Part model, mm, in its own coordinate system. A direction names the side the tool comes from. Give positions to 0.01 mm unless a question says otherwise; leave off trailing zeros. Order: outer loops, then holes, each group sorted by start corner. A loop starts at its lowest first (then second) coordinate and runs counter-clockwise, first axis right, second up. Notation, with made-up numbers: (87, -39.5) -> (125, -39.5) arc R19 cw to (125, -3.5) -> close; hole circle Ø1 at (-19.5, 22). An arc over 180 degrees is marked (long way). Write item = value, one per line. Start each with the question number.
Item 1: Band-saw the part on A-A on y = 37.5. Write the cut outline in (x, z), plus the area to 3 significant figures.
Item 2: Pull direction X, two halves, no side cores. Call faces 3 (the face through (0, 2, -20)), 4 (the face through (20, 2, -17)), 5 (the face through (-20, 2, 0)): +X half, -X half, draft (parallel to the pull), parting line (faces both ways), or undercut.
Item 3: Tool access for faces 1 (the face through (212.66, -0.648, 13.887)), 2 (the face through (420, 110, 0)): list every direction of +Z, -Z, +X, -X, +Y, -Y with a clear straight run to the whole face (end or side of a thin tool).
Item 4: Band-saw the part on B-B on z = 0. Write the cut outline in (x, y), plus the area to 3 significant figures.
Item 5: Flat gauge pins, fed straight in: P1, Ø6, axis at x = 295, z = 15, coming from the +Y side; P2, Ø8, axis at x = 155.5, y = 28, coming from the -Z side; P3, Ø1, axis at x = 66, z = 14, coming from the +Y side. Where does each tip first touch, or does it go through?
Item 6: Band-saw the part on D-D on x = 26. Write the cut outline in (y, z).
Item 7: Band-saw the part on C-C on y = 10. Write the cut outline in (x, z), plus the area to 3 significant figures.
Item 8: Drill centre lines: line 1 along X through (y, z) = (66.5, -0.5); line 2 along Y through (x, z) = (198, 10); line 3 along Y through (x, z) = (87, -11). Where is each one in solid material? Low to high.
```python
from build123d import *

# Parameters (mm, degrees)
SKETCH1_W           = 40
SKETCH1_H           = 40
BOSS_EXTRUDE1_DEPTH = 110
SKETCH2_R           = 17.5
BOSS_EXTRUDE2_DEPTH = 210


with BuildPart() as part:
    # Sketch1 → Boss-Extrude1 (new body, symmetric)
    with BuildSketch(Plane(origin=(0, 0, 0), x_dir=(1, 0, 0), z_dir=(0, 1, 0))):
        Rectangle(SKETCH1_W, SKETCH1_H)
    extrude(amount=BOSS_EXTRUDE1_DEPTH, both=True)

    # Sketch2 → Boss-Extrude2 (add)
    with BuildSketch(Plane(origin=(0, 0, 0), x_dir=(0, 0, -1), z_dir=(1, 0, 0))):
        with Locations((0, 10)):
            Circle(SKETCH2_R)
    extrude(amount=BOSS_EXTRUDE2_DEPTH)

    # Mirror7: part across plane


with BuildPart() as part_1:
    add(part.part)
    add(part.part.mirror(Plane(origin=(210, 10, 0), x_dir=(0, 0, 1), z_dir=(1, 0, 0))))


solid = part_1.part
```
Values found:
q1.outline = (-20, -20) -> (20, -20) -> (20, 20) -> (-20, 20) -> close; (400, -20) -> (440, -20) -> (440, 20) -> (400, 20) -> close
q1.area = 3,200 mm^2
q2.face_3 = draft
q2.face_4 = undercut
q2.face_5 = -X half
q3.face_1 = none
q3.face_2 = +Z, -Z, +X, -X, +Y
q4.outline = (-20, -110) -> (20, -110) -> (20, -7.5) -> (400, -7.5) -> (400, -110) -> (440, -110) -> (440, 110) -> (400, 110) -> (400, 27.5) -> (20, 27.5) -> (20, 110) -> (-20, 110) -> close
q4.area = 30,900 mm^2
q5.P1 = 22.74
q5.P2 = -10.5
q5.P3 = 21.14
q6.outline = circle Ø35 at (10, 0)
q7.outline = (-20, -20) -> (20, -20) -> (20, -17.5) -> (400, -17.5) -> (400, -20) -> (440, -20) -> (440, 20) -> (400, 20) -> (400, 17.5) -> (20, 17.5) -> (20, 20) -> (-20, 20) -> close
q7.area = 16,500 mm^2
q8.line_1 = -20 to 20, 400 to 440
q8.line_2 = -4.36 to 24.36
q8.line_3 = -3.61 to 23.61
